Work out the finished part from the listing and answer in its coordinate system (mm). A direction names the side the tool comes from. Coordinates: 2 decimals unless noted, no trailing zeros. Order: outer loops, then holes, each group sorted by start corner. A loop starts at its lowest first (then second) coordinate and runs counter-clockwise, first axis right, second up. Notation, with made-up numbers: (-1, -12.5) -> (9, -12.5) arc R28 ccw to (9, 14.5) -> close; hole circle Ø9 at (-7.5, 9.25). An arc over 180 degrees is marked (long way). Use one line per item in the form item = value.
from build123d import *

# Parameters (mm, degrees)
EXTRUDE_1_DEPTH        = 20
CUT_EXTRUDE_1_DEPTH    = 14.621320344
PATTERN_LINEAR_1_COUNT = 3
PATTERN_LINEAR_1_PITCH = 20


with BuildPart() as part:
    # Эскиз1 → Вытянуть-Тонкостенный1 (new body)
    with BuildSketch(Plane.XY):
        Polygon((-27.878679656, 14.142135624), (-13.736544033, 0), (13.736544033, 0), (27.878679656, 14.142135624), (30, 12.02081528), (14.97918472, -3), (-14.97918472, -3), (-30, 12.02081528), align=None)
    extrude(amount=EXTRUDE_1_DEPTH)

    # Эскиз2 → Вырез-Вытянуть1 (cut, through all)
    with BuildSketch(Plane(origin=(-6.868272016, -6.868272016, 0), x_dir=(0, 0, -1), z_dir=(0.707106781, 0.707106781, 0))):
        with BuildLine():
            Line((-7, 17.213203436), (-13, 17.213203436))
            ThreePointArc((-13, 17.213203436), (-15.5, 19.713203436), (-13, 22.213203436))
            Line((-13, 22.213203436), (-7, 22.213203436))
            ThreePointArc((-7, 22.213203436), (-4.5, 19.713203436), (-7, 17.213203436))
        make_face()
    cut_extrude_1 = extrude(amount=-CUT_EXTRUDE_1_DEPTH, mode=Mode.SUBTRACT)

    # Зеркальное отражение1: Вырез-Вытянуть1 across plane
    add(cut_extrude_1.mirror(Plane(origin=(0, 0, 0), x_dir=(0, 0, 1), z_dir=(1, 0, 0))), mode=Mode.SUBTRACT)


with BuildPart() as pattern_linear_1_1:
    # Линейный массив1: pattern copy
    add(part.part.moved(Location(Vector(0, 0, -1) * (1 * PATTERN_LINEAR_1_PITCH))))


with BuildPart() as pattern_linear_1_2:
    # Линейный массив1: pattern copy
    add(part.part.moved(Location(Vector(0, 0, -1) * (2 * PATTERN_LINEAR_1_PITCH))))


with BuildPart() as part_1:
    add(part.part)

    # Combine 2: union Линейный массив1_1, Линейный массив1_2
    add(pattern_linear_1_1.part)
    add(pattern_linear_1_2.part)


solid = part_1.part
(1) Each of these flat-tipped pins is pushed along its axis until it touches: P1, Ø8, axis at x = 14.5, z = -1, coming from the +Y side; P2, Ø5, axis at y = 10.5, z = -0.5, coming from the +X side; P3, Ø8, axis at x = -6.5, z = 2, coming from the +Y side. Where does it stop, or does it pass through?
Data:
P1 = 4.76
P2 = 30
P3 = 0
(2) Which of the six approach directions +Z, -Z, +X, -X, +Y, -Y give full straight-line access (tool end or side, diameter ignored) to faces 4 (the flat face through (0, 0, -10)), 5 (the flat face through (0, -1, -40)), 6 (the cylindrical face through (21.9, 6.1, -15.5)), 7 (the flat face through (-20.086, 4.257, -10.042)), 8 (the flat face through (-23.621, 7.793, -29.958))?
Data:
face_4 = +Z, -Z, +Y
face_5 = -Z, +X, -X, +Y, -Y
face_6 = none
face_7 = -X, +Y
face_8 = -Y
(3) Section A-A on z = -28.5 is taken. Write down the section's boundary in (x, y), plus the area to 3 significant figures.
Data:
outline = (-30, 12.02) -> (-24.7, 6.72) -> (-22.58, 8.84) -> (-27.88, 14.14) -> close; (-21.16, 3.18) -> (-14.98, -3) -> (14.98, -3) -> (21.16, 3.18) -> (19.04, 5.3) -> (13.74, 0) -> (-13.74, 0) -> (-19.04, 5.3) -> close; (22.58, 8.84) -> (24.7, 6.72) -> (30, 12.02) -> (27.88, 14.14) -> close
area = 180 mm²
(4) Section D-D on y = 6 is taken. Count the separate pieces of the cut face and the enclosed holes in it, plus the area to 3 significant figures.
Data:
separate_pieces = 8
enclosed_holes = 0
area = 237 mm²
(5) The mould has two halves that part along X. Classify faces 1 (the flat face through (-20.086, 4.257, -30.042)), 2 (the flat face through (28.92, 13.1, -10.42)), 3 (the flat face through (-23.621, 7.793, 10.042)): released by +X, released by -X, zero draft, split by the parting line, or undercut.
Data:
face_1 = released by -X
face_2 = released by +X
face_3 = undercut
(6) Straight lines are drawn through the part: line 1 along Y through (x, z) = (2.5, -9); line 2 along X through (y, z) = (6.75, -14); line 3 along X through (y, z) = (8.5, 17.5). For each, find the intervals that lie inside material, in ascending order.
Data:
line_1 = -3 to 0
line_2 = -24.73 to -24.37, 24.37 to 24.73
line_3 = -26.48 to -22.24, 22.24 to 26.48
(7) Section C-C on x = -11 is taken. Write down the section's boundary in (y, z).
Data:
outline = (-3, -40) -> (0, -40) -> (0, 20) -> (-3, 20) -> close
(8) Section B-B on z = -2 is taken. Write down the section's boundary in (x, y).
Data:
outline = (-30, 12.02) -> (-14.98, -3) -> (14.98, -3) -> (30, 12.02) -> (27.88, 14.14) -> (13.74, 0) -> (-13.74, 0) -> (-27.88, 14.14) -> close
